Autodesk Inventor part; units mm, degrees
ref_plane "Arbeitsebene1" through (-29, 0, 0) normal (1, 0, 0) x (0, 1, 0)
ref_plane "Arbeitsebene2" through (0, 0, -44.5) normal (0, 0, 1) x (1, 0, 0)
ref_plane "XZ Plane" through (0, 0, 0) normal (0, 1, 0) x (-1, 0, 0)
sketch "Skizze1" plane through (0, 0, 0) normal (0, 1, 0) x (-1, 0, 0)
  line L0 (0, 0) -> (58, 0)
  line L1 (58, 0) -> (58, -89)
  arc A0 (58, -89) -> (48.5, -98.5) centre (58, -98.5) ccw
  line L2 (48.5, -98.5) -> (48.5, -218.5)
  line L3 (48.5, -218.5) -> (48.5, -234.2814)
  line L4 (0, 0) -> (0, -395.7321)
  line L5 (48.5, -218.5) -> (48.5, -250.0629) construction
  arc A1 (0, -395.7321) -> (1.4803, -399.6783) centre (6, -395.7321) ccw
  line L6 (1.4803, -399.6783) -> (7, -406)
  line L7 (7, -406) -> (29, -367.8949)
  line L8 (29, -367.8949) -> (29, -367.8949)
  arc A2 (24.7603, -358.6329) -> (29, -367.8949) centre (33.3956, -360.2814) ccw
  line L9 (24.7603, -358.6329) -> (48.5, -234.2814)
  line L10 (7, -406) -> (55.5885, -321.8422) construction
  dimension "d1" = 58
  dimension "d2" = 9.5
  dimension "d3" = 89
  dimension "d4" = 120
  dimension "d7" = 406
  dimension "d8" = 44
  dimension "d9" = 30
  dimension "d10" = 6
  dimension "d11" = 126
  dimension "d12" = 29
  dimension "d13" = 6
extrude "Extrusion1" add sketch "Skizze1" along normal blind 6
sketch "Skizze2" plane through (0, 6, 0) normal (0, 1, 0) x (1, 0, 0)
  line L0 (-46, 12) -> (-12, 12)
  line L1 (-12, 12) -> (-12, 77)
  line L2 (-12, 77) -> (-46, 77)
  line L3 (-46, 77) -> (-46, 12)
  line L4 (-58, 0) -> (0, 0)
  point P0 (-29, 12)
  point P1 (-29, 0)
  dimension "d16" = 34
  dimension "d17" = 65
  dimension "d18" = 12
extrude "Extrusion2" cut sketch "Skizze2" against normal up to surface (6 mm away)
sketch "Skizze3" plane through (0, 6, 0) normal (0, 1, 0) x (1, 0, 0)
  line L0 (-58, 0) -> (0, 0)
  point P0 (-40, 5)
  point P1 (-18, 5)
  point P2 (-29, 0)
  point P3 (-29, 0)
  dimension "d21" = 11
  dimension "d22" = 11
  dimension "d23" = 5
hole "Bohrung1" at (-40, 6, -5) at (-18, 6, -5) direction (0, -1, 0) diameter 5 end through all
sketch "Skizze4" plane through (0, 6, 0) normal (0, 1, 0) x (1, 0, 0)
  circle A0 centre (-40, 5) radius 2.5
  line L0 (-58, 89) -> (-58, 0)
  point P0 (0, 0)
  point P1 (-52, 15)
  point P2 (-52, 34)
  point P3 (-52, 53)
  point P4 (-52, 72)
  dimension "d31" = 10
  dimension "d32" = 19
  dimension "d33" = 19
  dimension "d34" = 19
  dimension "d35" = 6
hole "Bohrung2" at (-52, 6, -15) at (-52, 6, -34) at (-52, 6, -53) at (-52, 6, -72) direction (0, -1, 0) diameter 5 depth 6
ref_plane "Arbeitsebene1" through (-29, 0, 0) normal (1, 0, 0) x (0, 1, 0)
mirror "Spiegeln1" about plane through (-29, 0, 0) normal (1, 0, 0) of "Bohrung2"
ref_plane "Arbeitsebene2" through (0, 0, -44.5) normal (0, 0, 1) x (1, 0, 0)
mirror "Spiegeln2" about plane through (0, 0, -44.5) normal (0, 0, 1) of "Bohrung1"
sketch "Skizze5" plane through (0, 6, 0) normal (0, 1, 0) x (1, 0, 0)
  circle A0 centre (-18, 84) radius 2.5
  line L0 (0, 0) -> (0, 395.7321)
  point P0 (-10, 103)
  point P1 (-10, 132)
  point P2 (-10, 161)
  point P3 (-10, 190)
  point P4 (-10, 277)
  point P5 (-10, 306)
  point P6 (-10, 335)
  point P7 (-10, 219)
  point P8 (-10, 248)
  dimension "d45" = 19
  dimension "d46" = 29
  dimension "d47" = 29
  dimension "d48" = 29
  dimension "d49" = 29
  dimension "d50" = 29
  dimension "d51" = 29
  dimension "d52" = 29
  dimension "d53" = 29
  dimension "d54" = 10
hole "Bohrung3" at (-10, 6, -103) at (-10, 6, -132) at (-10, 6, -161) at (-10, 6, -190) at (-10, 6, -277) at (-10, 6, -306) at (-10, 6, -335) at (-10, 6, -219) at (-10, 6, -248) direction (0, -1, 0) diameter 5 depth 6
sketch "Skizze6" plane through (0, 6, 0) normal (0, 1, 0) x (1, 0, 0)
  arc A0 (-58, 89) -> (-48.5, 98.5) centre (-58, 98.5) ccw
  line L0 (-48.5, 234.2814) -> (-48.5, 98.5)
  point P0 (0, 0)
  point P1 (-41.5, 149.5)
  point P2 (-41.5, 174.5)
  point P3 (-41.5, 212.5)
  dimension "d62" = 51
  dimension "d63" = 25
  dimension "d64" = 38
  dimension "d65" = 7
hole "Bohrung4" at (-41.5, 6, -149.5) at (-41.5, 6, -174.5) at (-41.5, 6, -212.5) direction (0, -1, 0) diameter 5 depth 6
sketch "Skizze8" plane through (0, 6, 0) normal (0, 1, 0) x (1, 0, 0)
  line L0 (-7, 406) -> (-29, 367.8949)
  line L1 (-4.2402, 402.8391) -> (-26.0353, 365.0889) construction
  arc A0 (-24.7603, 358.6329) -> (-29, 367.8949) centre (-33.3956, 360.2814) ccw
  line L2 (-1.4803, 399.6783) -> (-7, 406)
  line L3 (-15.1377, 383.964) -> (-49.9282, 404.0503) construction
  line L4 (-22.1377, 371.8397) -> (-7.4153, 363.3397) construction
  point P0 (0, 0)
  point P1 (-8.1377, 396.0884)
  dimension "d90" = 90
  dimension "d91" = 14
  dimension "d92" = 28
  dimension "d93" = 90
  dimension "d94" = 17
hole "Bohrung5" at (-7.4153, 6, -363.3397) at (-22.1377, 6, -371.8397) at (-8.1377, 6, -396.0884) direction (0, -1, 0) diameter 4.917 depth 6
properties part number "1012"
Geometry check sheet. Reference: the model listing, model coordinates, mm. A direction names the side the tool comes from. Coordinates: 2 decimals unless noted, no trailing zeros. Write each loop counter-clockwise with the first axis right and the second up, starting at its lowest first coordinate (ties: lowest second). Pieces come first, ordered by that corner, then holes. Notation, with made-up numbers: M -31.5,9 L 4.5,9 A23 cw 4.5,43 Z; hole C 44,86 d8. An arc over 180 degrees is marked long. Answer as a JSON object with one key per item and string values.
1. Section check B-B, the plane z = -378.5. Enter the section's corners in (x, y).
Answers below:
{"outline": "M -22.88,0 L 0,0 L 0,6 L -22.88,6 Z"}
2. Section check A-A, the plane y = 2.75. Give the number of separate pieces and of enclosed holes in the cut face, plus the area to 3 significant figures.
Answers below:
{"separate pieces": "1", "enclosed holes": "28", "area": "14,900 mm²"}
3. Section check C-C, the plane z = -266.5. Enter the section's corners in (x, y).
Answers below:
{"outline": "M -42.35,0 L 0,0 L 0,6 L -42.35,6 Z"}
4. Tool access check on faces 1 (the flat face through (-36.464, 2.958, -297.328)), 2 (the flat face through (-22, 0, -200)). Record the directions out of +Z, -Z, +X, -X, +Y, -Y that give a thin tool (end or side, any length) a straight path to the whole face; none if there is none.
Answers below:
{"face 1": "-X, +Y, -Y", "face 2": "+Z, -Z, +X, -X, -Y"}
5. Scan lines: L1, parallel to X at y = 4.5, z = -53; L2, parallel to X at y = 4.25, z = -84; L3, parallel to X at y = 2.7, z = -60.5. Record each from-to range of solid material in increasing order.
Answers below:
{"L1": "x = -58 to -54.5, -49.5 to -46, -12 to -8.5, -3.5 to 0", "L2": "x = -58 to -42.5, -37.5 to -20.5, -15.5 to 0", "L3": "x = -58 to -46, -12 to 0"}
6. Go/stop test with flat-tipped pins: pin 1 Ø3 at (x, z) = (-40, -84) entering from -Y; pin 2 Ø2 at (y, z) = (3, -329) entering from -X; pin 3 Ø1.5 at (y, z) = (4, -187) entering from -X; pin 4 Ø2 at (x, y) = (-7.5, 2) entering from -Z. Record where each tip stops, or that it passes through.
Answers below:
{"pin 1": "passes through", "pin 2": "stops at x = -30.61", "pin 3": "stops at x = -48.5", "pin 4": "stops at z = -406"}
